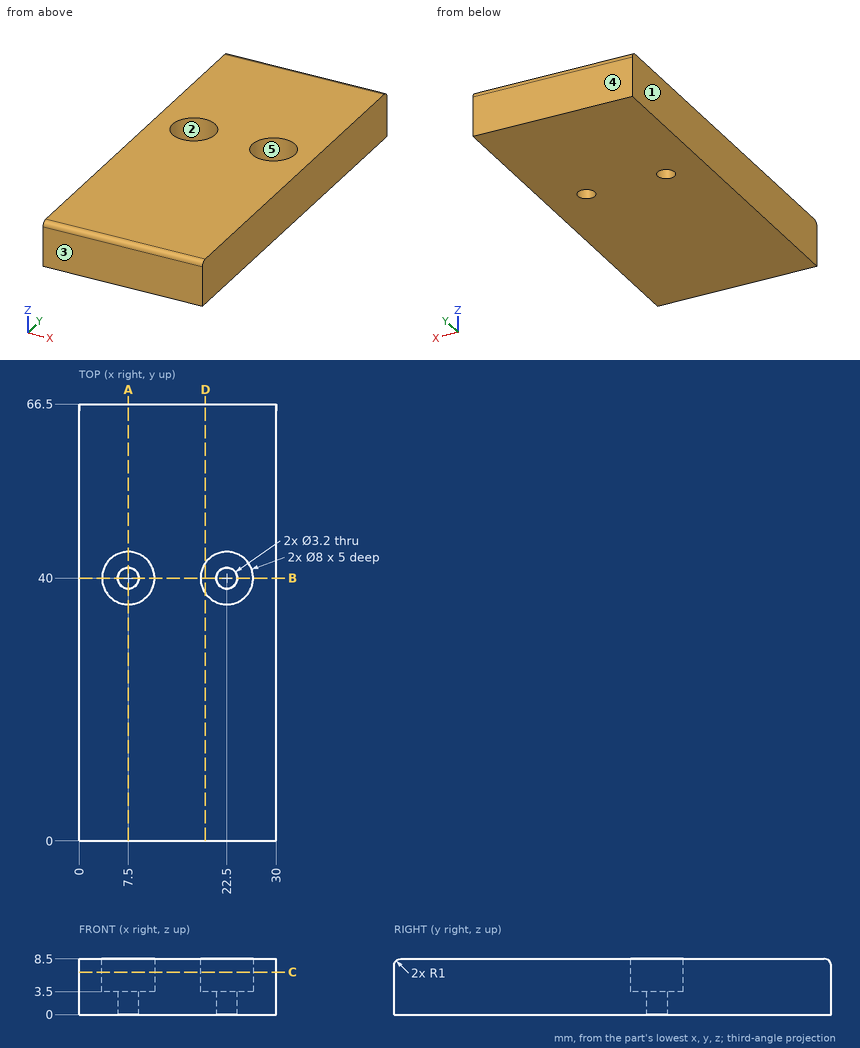
For this review, use the dimensioned drawing (mm, ordinates from the lowest corner) and the shaded views. A direction names the side the tool comes from. Coordinates: 2 decimals unless noted, no trailing zeros. Order: outer loops, then holes, each group sorted by start corner. A loop starts at its lowest first (then second) coordinate and runs counter-clockwise, first axis right, second up. Notation, with made-up numbers: M 55,-9 L 107,-9 A17 cw 107,16 Z; hole C -27.75,34 d7. An arc over 180 degrees is marked long. Answer as a JSON object with one key per item and string values. Group by question number.
1) Add section B-B, the plane y = 40. Write out the cut boundary in (x, z), then the cut area to 3 significant figures.
2) Mouldability with a two-part tool opening along Y and no side actions: class the marked faces 1, 2 and 3 as pulls with the +Y half, pulls with the -Y half, needs draft (parallel to the pull), parting line crosses it, or undercut.
3) Wall thickness on L1, parallel to Y at x = 7.5, z = 1.2; L2, parallel to Y at x = 19.25, z = 4; L3, parallel to Z at x = 20, y = 40: over which ranges is each line inside the solid? List them lowest first.
4) For pin 1 (2.5 mm diameter, centred on x = 22, y = 39.5, fed in from +Z); pin 2 (5 mm diameter, centred on x = 7.5, y = 40, fed in from -Z), all flat-tipped, find the tip position at first contact; note any pin that passes through.
5) Add section D-D, the plane x = 19.25. Write out the cut boundary in (y, z), then the cut area to 3 significant figures.
6) Add section A-A, the plane x = 7.5. Write out the cut boundary in (y, z), then the cut area to 3 significant figures.
7) Add section C-C, the plane z = 6.5. Write out the cut boundary in (x, y).
8) Tool access review of the marked faces 4 and 5: name each direction out of +Z, -Z, +X, -X, +Y, -Y from which nothing blocks a thin tool from reaching the whole face with its end or side.
Computed values:
{
 "1": {"outline": "M 0,0 L 5.9,0 L 5.9,3.5 L 3.5,3.5 L 3.5,8.5 L 0,8.5 Z; M 9.1,0 L 20.9,0 L 20.9,3.5 L 18.5,3.5 L 18.5,8.5 L 11.5,8.5 L 11.5,3.5 L 9.1,3.5 Z; M 24.1,0 L 30,0 L 30,8.5 L 26.5,8.5 L 26.5,3.5 L 24.1,3.5 Z", "area": "153 mm^2"},
 "2": {"face 1": "needs draft", "face 2": "undercut", "face 3": "pulls with the -Y half"},
 "3": {"L1": "y = 0 to 38.4, 41.6 to 66.5", "L2": "y = 0 to 37.67, 42.33 to 66.5", "L3": "z = 0 to 3.5"},
 "4": {"pin 1": "stops at z = 3.5", "pin 2": "stops at z = 0"},
 "5": {"outline": "M 0,0 L 66.5,0 L 66.5,7.5 A1 ccw 65.5,8.5 L 42.33,8.5 L 42.33,3.5 L 37.67,3.5 L 37.67,8.5 L 1,8.5 A1 ccw 0,7.5 Z", "area": "542 mm^2"},
 "6": {"outline": "M 0,0 L 38.4,0 L 38.4,3.5 L 36,3.5 L 36,8.5 L 1,8.5 A1 ccw 0,7.5 Z; M 41.6,0 L 66.5,0 L 66.5,7.5 A1 ccw 65.5,8.5 L 44,8.5 L 44,3.5 L 41.6,3.5 Z", "area": "514 mm^2"},
 "7": {"outline": "M 0,0 L 30,0 L 30,66.5 L 0,66.5 Z; hole C 7.5,40 d8; hole C 22.5,40 d8"},
 "8": {"face 4": "+Z, -Z, +X, -X, +Y", "face 5": "+Z"}
}
